Geometry: final body of the model. Coordinates: model frame, mm. A direction names the side the tool comes from. Give positions to 0.01 mm unless a question says otherwise; leave off trailing zeros. Order: outer loops, then holes, each group sorted by start corner. A loop starts at its lowest first (then second) coordinate and runs counter-clockwise, first axis right, second up. Notation, with made-up numbers: (41, -23) -> (50, -23) arc R22 ccw to (50, -11) -> close; hole circle Ø3 at (69, -29.5). An arc over 180 degrees is marked (long way). One line per question, with ' | ' between items. Start each with the question number.
(1) Section B-B (y = 90). Return loops of the section in (x, z), then the cut area to 3 significant figures.
(2) Mould query, pull axis Y, two halves, no side actions, for faces 5 (the face through (7.89, -13.92, 2.96)), 6 (the face through (181, 9, 3)), 7 (the face through (-2.41, 44.59, 2.96)). Classes: +Y half, -Y half, draft (parallel to the pull), parting line (faces both ways), or undercut.
(3) Section D-D (y = 30.5). Return loops of the section in (x, z).
(4) Section C-C (z = 2.75). State how many separate pieces and enclosed holes the cut face has, then the cut area to 3 significant figures.
(5) Set-up query: faces 1 (the face through (135.19, 20.96, 2.96)), 2 (the face through (186.42, 70.68, 2.96)), 3 (the face through (0, 85, 3)), 4 (the face through (24.11, 96.93, 2.96)). Return all of +Z, -Z, +X, -X, +Y, -Y with unobstructed straight access to the full face (end or side cutting, diameter ignored); none if empty.
(6) Section A-A (x = 167.5). Return loops of the section in (y, z), then the cut area to 3 significant figures.
(7) Ray query, L1, parallel to Y at x = 64, z = 1.3; L2, parallel to Y at x = 79.5, z = 0.4; L3, parallel to Y at x = 41, z = 1.1. Return the intervals inside material, ascending.
```python
from build123d import *

# Parameters (mm, degrees)
F0_R     = 11.1
F0_R_2   = 1.5
F1_DEPTH = 6
F2_DEPTH = 6


# Not quite as in the source:
# - a feature names something its author has since deleted; it is built from what else it names


with BuildPart() as f1:
    # F0 (on Top) → F1 (new body)
    with BuildSketch(Plane.XY):
        Polygon((32, 18.4752086141), (16, 9.237604307), (16, -9.237604307), (32, -18.4752086141), (48, -9.237604307), (48, 9.237604307), align=None)
        with Locations((32, 0)):
            Circle(F0_R, mode=Mode.SUBTRACT)
        Polygon((16, -9.237604307), (16, 9.237604307), (0, 18.4752086141), (-2.5, 17.0318329411), (-5, 15.5884572681), (-16, 9.237604307), (-16, -9.237604307), (0, -18.4752086141), align=None)
        Circle(F0_R, mode=Mode.SUBTRACT)
        Polygon((0, 18.4752086141), (16, 9.237604307), (32, 18.4752086141), (32, 36.9504172281), (16, 46.1880215352), (0, 36.9504172281), (0, 22.805335633), (0, 21.36195996), align=None)
        with Locations((16, 27.7128129211)):
            Circle(F0_R, mode=Mode.SUBTRACT)
        Polygon((-2.5, 17.0318329411), (0, 18.4752086141), (0, 21.36195996), (-2.5, 22.805335633), (-5, 21.36195996), (-5, 18.4752086141), align=None)
        with Locations((-2.5, 19.918584287)):
            Circle(F0_R_2, mode=Mode.SUBTRACT)
        Polygon((32, 36.9504172281), (32, 18.4752086141), (48, 9.237604307), (64, 18.4752086141), (64, 36.9504172281), (48, 46.1880215352), align=None)
        with Locations((48, 27.7128129211)):
            Circle(F0_R, mode=Mode.SUBTRACT)
        Polygon((64, 18.4752086141), (48, 9.237604307), (48, -9.237604307), (64, -18.4752086141), (80, -9.237604307), (80, 9.237604307), align=None)
        with Locations((64, 0)):
            Circle(F0_R, mode=Mode.SUBTRACT)
        Polygon((16, 46.1880215352), (32, 36.9504172281), (48, 46.1880215352), (48, 64.6632301492), (32, 73.9008344563), (16, 64.6632301492), align=None)
        with Locations((32, 55.4256258422)):
            Circle(F0_R, mode=Mode.SUBTRACT)
        Polygon((64, 36.9504172281), (64, 18.4752086141), (80, 9.237604307), (96, 18.4752086141), (96, 36.9504172281), (80, 46.1880215352), align=None)
        with Locations((80, 27.7128129211)):
            Circle(F0_R, mode=Mode.SUBTRACT)
        Polygon((0, 36.9504172281), (16, 46.1880215352), (16, 64.6632301492), (0, 73.9008344563), (-2.5, 72.4574587833), (-5, 71.0140831103), (-16, 64.6632301492), (-16, 46.1880215352), align=None)
        with Locations((0, 55.4256258422)):
            Circle(F0_R, mode=Mode.SUBTRACT)
        Polygon((48, 64.6632301492), (48, 46.1880215352), (64, 36.9504172281), (80, 46.1880215352), (80, 64.6632301492), (64, 73.9008344563), align=None)
        with Locations((64, 55.4256258422)):
            Circle(F0_R, mode=Mode.SUBTRACT)
        Polygon((96, 18.4752086141), (80, 9.237604307), (80, -9.237604307), (96, -18.4752086141), (112, -9.237604307), (112, 9.237604307), align=None)
        with Locations((96, 0)):
            Circle(F0_R, mode=Mode.SUBTRACT)
        Polygon((32, 73.9008344563), (48, 64.6632301492), (64, 73.9008344563), (64, 92.3760430703), (48, 101.6136473774), (32, 92.3760430703), align=None)
        with Locations((48, 83.1384387633)):
            Circle(F0_R, mode=Mode.SUBTRACT)
        Polygon((96, 36.9504172281), (96, 18.4752086141), (112, 9.237604307), (128, 18.4752086141), (128, 36.9504172281), (112, 46.1880215352), align=None)
        with Locations((112, 27.7128129211)):
            Circle(F0_R, mode=Mode.SUBTRACT)
        Polygon((80, 64.6632301492), (80, 46.1880215352), (96, 36.9504172281), (112, 46.1880215352), (112, 64.6632301492), (96, 73.9008344563), align=None)
        with Locations((96, 55.4256258422)):
            Circle(F0_R, mode=Mode.SUBTRACT)
        Polygon((-2.5, 72.4574587833), (0, 73.9008344563), (0, 76.7875858022), (-2.5, 78.2309614752), (-5, 76.7875858022), (-5, 73.9008344563), align=None)
        with Locations((-2.5, 75.3442101292)):
            Circle(F0_R_2, mode=Mode.SUBTRACT)
        Polygon((64, 92.3760430703), (64, 73.9008344563), (80, 64.6632301492), (96, 73.9008344563), (96, 92.3760430703), (80, 101.6136473774), align=None)
        with Locations((80, 83.1384387633)):
            Circle(F0_R, mode=Mode.SUBTRACT)
        Polygon((128, 18.4752086141), (112, 9.237604307), (112, -9.237604307), (128, -18.4752086141), (144, -9.237604307), (144, 9.237604307), align=None)
        with Locations((128, 0)):
            Circle(F0_R, mode=Mode.SUBTRACT)
        Polygon((128, 36.9504172281), (128, 18.4752086141), (144, 9.237604307), (160, 18.4752086141), (160, 36.9504172281), (144, 46.1880215352), align=None)
        with Locations((144, 27.7128129211)):
            Circle(F0_R, mode=Mode.SUBTRACT)
        Polygon((112, 64.6632301492), (112, 46.1880215352), (128, 36.9504172281), (144, 46.1880215352), (144, 64.6632301492), (128, 73.9008344563), align=None)
        with Locations((128, 55.4256258422)):
            Circle(F0_R, mode=Mode.SUBTRACT)
        Polygon((96, 92.3760430703), (96, 73.9008344563), (112, 64.6632301492), (128, 73.9008344563), (128, 92.3760430703), (112, 101.6136473774), align=None)
        with Locations((112, 83.1384387633)):
            Circle(F0_R, mode=Mode.SUBTRACT)
        Polygon((160, 18.4752086141), (144, 9.237604307), (144, -9.237604307), (160, -18.4752086141), (176, -9.237604307), (176, 4.9074772881), (176, 6.3508529611), (176, 9.237604307), align=None)
        with Locations((160, 0)):
            Circle(F0_R, mode=Mode.SUBTRACT)
        Polygon((160, 36.9504172281), (160, 18.4752086141), (176, 9.237604307), (178.5, 10.68097998), (181, 12.124355653), (192, 18.4752086141), (192, 36.9504172281), (176, 46.1880215352), align=None)
        with Locations((176, 27.7128129211)):
            Circle(F0_R, mode=Mode.SUBTRACT)
        Polygon((144, 64.6632301492), (144, 46.1880215352), (160, 36.9504172281), (176, 46.1880215352), (176, 60.3331031303), (176, 61.7764788033), (176, 64.6632301492), (160, 73.9008344563), align=None)
        with Locations((160, 55.4256258422)):
            Circle(F0_R, mode=Mode.SUBTRACT)
        Polygon((128, 92.3760430703), (128, 73.9008344563), (144, 64.6632301492), (160, 73.9008344563), (160, 92.3760430703), (144, 101.6136473774), align=None)
        with Locations((144, 83.1384387633)):
            Circle(F0_R, mode=Mode.SUBTRACT)
        Polygon((160, 92.3760430703), (160, 73.9008344563), (176, 64.6632301492), (178.5, 66.1066058222), (181, 67.5499814952), (192, 73.9008344563), (192, 92.3760430703), (176, 101.6136473774), align=None)
        with Locations((176, 83.1384387633)):
            Circle(F0_R, mode=Mode.SUBTRACT)
    extrude(amount=F1_DEPTH)

    # F0 (on Top) → F2 (join)
    with BuildSketch(Plane.XY):
        Polygon((0, 18.4752086141), (16, 9.237604307), (32, 18.4752086141), (32, 36.9504172281), (16, 46.1880215352), (0, 36.9504172281), (0, 22.805335633), (0, 21.36195996), align=None)
        with Locations((16, 27.7128129211)):
            Circle(F0_R, mode=Mode.SUBTRACT)
        Polygon((0, 73.9008344563), (16, 64.6632301492), (32, 73.9008344563), (32, 92.3760430703), (16, 101.6136473774), (0, 92.3760430703), (0, 78.2309614752), (0, 76.7875858022), align=None)
        with Locations((16, 83.1384387633)):
            Circle(F0_R, mode=Mode.SUBTRACT)
        Polygon((178.5, 10.68097998), (176, 9.237604307), (176, 6.3508529611), (178.5, 4.9074772881), (181, 6.3508529611), (181, 9.237604307), align=None)
        with Locations((178.5, 7.7942286341)):
            Circle(F0_R_2, mode=Mode.SUBTRACT)
        Polygon((178.5, 66.1066058222), (176, 64.6632301492), (176, 61.7764788033), (178.5, 60.3331031303), (181, 61.7764788033), (181, 64.6632301492), align=None)
        with Locations((178.5, 63.2198544763)):
            Circle(F0_R_2, mode=Mode.SUBTRACT)
        Polygon((-5, 71.0140831103), (-2.5, 72.4574587833), (-5, 73.9008344563), align=None)
        Polygon((-2.5, 78.2309614752), (0, 76.7875858022), (0, 78.2309614752), align=None)
        Polygon((-2.5, 22.805335633), (0, 21.36195996), (0, 22.805335633), align=None)
        Polygon((-5, 15.5884572681), (-2.5, 17.0318329411), (-5, 18.4752086141), align=None)
        Polygon((176, 61.7764788033), (176, 60.3331031303), (178.5, 60.3331031303), align=None)
        Polygon((181, 67.5499814952), (178.5, 66.1066058222), (181, 64.6632301492), align=None)
        Polygon((178.5, 4.9074772881), (176, 6.3508529611), (176, 4.9074772881), align=None)
        Polygon((181, 12.124355653), (178.5, 10.68097998), (181, 9.237604307), align=None)
    extrude(amount=F2_DEPTH)


solid = f1.part
```
Response:
1) outline: (0, 0) -> (7.27, 0) -> (7.27, 6) -> (0, 6) -> close; (24.73, 0) -> (39.27, 0) -> (39.27, 6) -> (24.73, 6) -> close; (56.73, 0) -> (71.27, 0) -> (71.27, 6) -> (56.73, 6) -> close; (88.73, 0) -> (103.27, 0) -> (103.27, 6) -> (88.73, 6) -> close; (120.73, 0) -> (135.27, 0) -> (135.27, 6) -> (120.73, 6) -> close; (152.73, 0) -> (167.27, 0) -> (167.27, 6) -> (152.73, 6) -> close; (184.73, 0) -> (192, 0) -> (192, 6) -> (184.73, 6) -> close | area: 524 mm^2
2) face 5: -Y half | face 6: draft | face 7: undercut
3) outline: (0, 0) -> (5.26, 0) -> (5.26, 6) -> (0, 6) -> close; (26.74, 0) -> (37.26, 0) -> (37.26, 6) -> (26.74, 6) -> close; (58.74, 0) -> (69.26, 0) -> (69.26, 6) -> (58.74, 6) -> close; (90.74, 0) -> (101.26, 0) -> (101.26, 6) -> (90.74, 6) -> close; (122.74, 0) -> (133.26, 0) -> (133.26, 6) -> (122.74, 6) -> close; (154.74, 0) -> (165.26, 0) -> (165.26, 6) -> (154.74, 6) -> close; (186.74, 0) -> (192, 0) -> (192, 6) -> (186.74, 6) -> close
4) separate pieces: 1 | enclosed holes: 28 | area: 12,100 mm^2
5) face 1: +Z, -Z | face 2: +Z, -Z, +X | face 3: +Z, -Z, -X, +Y | face 4: +Z, -Z, +Y
6) outline: (-14.15, 0) -> (-8.18, 0) -> (-8.18, 6) -> (-14.15, 6) -> close; (8.18, 0) -> (20.57, 0) -> (20.57, 6) -> (8.18, 6) -> close; (34.85, 0) -> (47.24, 0) -> (47.24, 6) -> (34.85, 6) -> close; (63.61, 0) -> (76, 0) -> (76, 6) -> (63.61, 6) -> close; (90.28, 0) -> (96.71, 0) -> (96.71, 6) -> (90.28, 6) -> close | area: 297 mm^2
7) L1: y = -18.48 to -11.1, 11.1 to 44.33, 66.53 to 92.38 | L2: y = -9.53 to 16.62, 38.8 to 72.05, 94.23 to 101.32 | L3: y = -13.28 to -6.5, 6.5 to 19.1, 36.33 to 48.93, 61.92 to 74.52, 91.75 to 97.57
